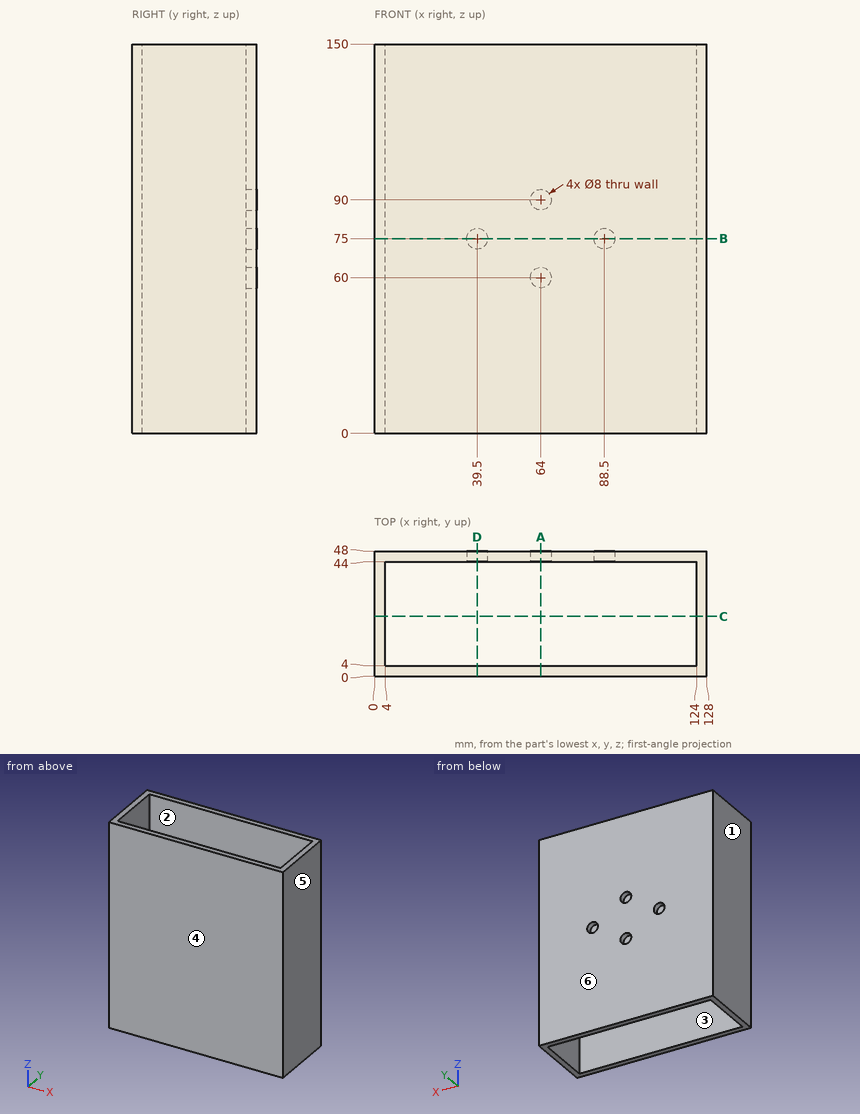
The drawing under review shows one solid part. Ordinate dimensions are in mm from its lowest x, y, z. A direction names the side the tool comes from. Give positions to 0.01 mm unless a question says otherwise; leave off trailing zeros. Write each loop counter-clockwise with the first axis right and the second up, starting at its lowest first coordinate (ties: lowest second). Pieces come first, ordered by that corner, then holes. Notation, with made-up numbers: (73.25, 5) - (129.25, 5) arc R20 cw to (129.25, 12) - close; hole circle Ø2 at (-20, 70). An arc over 180 degrees is marked (long way). Answer in a Markdown table with one row per item. Add a question column.
1. We need section C-C on y = 23. Write out the cut boundary in (x, z), then the cut area to 3 significant figures.
2. Tool access review of the marked faces 1 and 2: name each direction out of +Z, -Z, +X, -X, +Y, -Y from which nothing blocks a thin tool from reaching the whole face with its end or side.
3. Draft analysis for pull direction Y (two halves, no side actions). For the marked faces 3, 4, 5 and 6, state which applies: +Y half, -Y half, draft (parallel to the pull), parting line (faces both ways), or undercut.
4. We need section D-D on x = 39.5. Write out the cut boundary in (y, z), then the cut area to 3 significant figures.
5. We need section B-B on z = 75. Write out the cut boundary in (x, y), then the cut area to 3 significant figures.
6. Wall thickness on line 1 along Y through (x, z) = (57.5, 35); line 2 along Z through (x, y) = (64, 45); line 3 along X through (y, z) = (17.5, 25): over which ranges is each line inside the solid? List them lowest first. Write a range as [from, to].
7. We need section A-A on x = 64. Write out the cut boundary in (y, z), then the cut area to 3 significant figures.
Ans:
| question | item | result |
|---|---|---|
| 1 | outline | (0, 0) - (4, 0) - (4, 150) - (0, 150) - close; (124, 0) - (128, 0) - (128, 150) - (124, 150) - close |
| 1 | area | 1,200 mm^2 |
| 2 | face 1 | +Z, -Z, -X, +Y, -Y |
| 2 | face 2 | +Z, -Z |
| 3 | face 3 | undercut |
| 3 | face 4 | -Y half |
| 3 | face 5 | draft |
| 3 | face 6 | +Y half |
| 4 | outline | (0, 0) - (4, 0) - (4, 150) - (0, 150) - close; (44, 0) - (48, 0) - (48, 71) - (44, 71) - close; (44, 79) - (48, 79) - (48, 150) - (44, 150) - close |
| 4 | area | 1,170 mm^2 |
| 5 | outline | (0, 0) - (128, 0) - (128, 48) - (92.5, 48) - (92.5, 44) - (124, 44) - (124, 4) - (4, 4) - (4, 44) - (35.5, 44) - (35.5, 48) - (0, 48) - close; (43.5, 44) - (84.5, 44) - (84.5, 48) - (43.5, 48) - close |
| 5 | area | 1,280 mm^2 |
| 6 | line 1 | y = [0, 4], [44, 48] |
| 6 | line 2 | z = [0, 56], [64, 86], [94, 150] |
| 6 | line 3 | x = [0, 4], [124, 128] |
| 7 | outline | (0, 0) - (4, 0) - (4, 150) - (0, 150) - close; (44, 0) - (48, 0) - (48, 56) - (44, 56) - close; (44, 64) - (48, 64) - (48, 86) - (44, 86) - close; (44, 94) - (48, 94) - (48, 150) - (44, 150) - close |
| 7 | area | 1,140 mm^2 |
